Verification items for the finished model (mm, model axes). Give positions to 0.01 mm unless a question says otherwise; leave off trailing zeros. Write each loop counter-clockwise with the first axis right and the second up, starting at its lowest first coordinate (ties: lowest second). Pieces come first, ordered by that corner, then holes. Notation, with made-up numbers: M 25.5,78 L 35.5,78 A16 cw 35.5,98 Z; hole C -9.75,59.25 d7. An arc over 180 degrees is marked long. Write item = value, one per line.
from build123d import *

# Parameters (mm, degrees)
SKETCH3_W = 9
SKETCH3_H = 1.5


with BuildPart() as part:
    # Sweep1: sweep along a path in Sketch2
    with BuildLine(Plane.XY.offset(-150.483366658)) as sweep1_path:
        Line((-1, 148.379342702), (883.52063783, 148.379342702))
        ThreePointArc((883.52063783, 148.379342702), (890.42063783, 141.479342703), (883.52063783, 134.579342702))
        Line((883.52063783, 134.579342702), (-1, 134.579342702))
        ThreePointArc((-1, 134.579342702), (-7.9, 141.479342702), (-1, 148.379342702))
    # Sketch3 → Sweep1 (sweep)
    with BuildSketch(Plane(origin=(0, 0, 0), x_dir=(0, 0, -1), z_dir=(1, 0, 0))):
        with Locations((145.983366658, 147.629342702)):
            Rectangle(SKETCH3_W, SKETCH3_H)
    sweep(path=sweep1_path.line)


solid = part.part
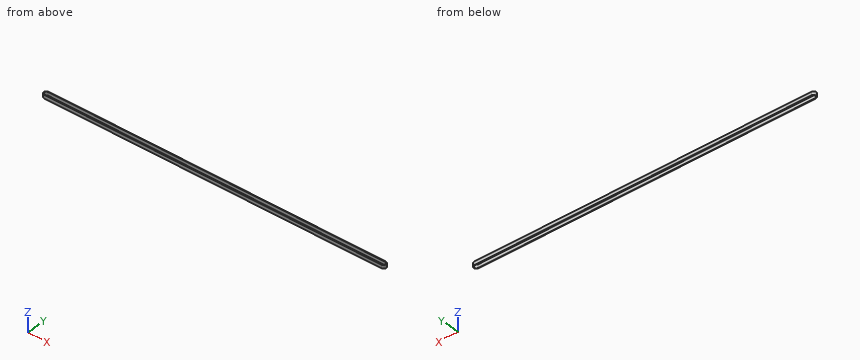
1) Depth check by flat-ended pin: P1, Ø1.5, axis at y = 142.5, z = -149.5, coming from the +X side; P2, Ø3, axis at y = 137, z = -147.5, coming from the -X side; P3, Ø1, axis at y = 146, z = -143.5, coming from the -X side. Enter the tip coordinate at first touch or a pass-through.
From the geometry:
P1 = 890.42
P2 = -7.22
P3 = -6.61
2) Cross-section at B-B on z = -145.5. Record the boundary of the cut face in (x, y).
From the geometry:
outline = M -1,134.58 L 883.52,134.58 A6.9 ccw 883.52,148.38 L -1,148.38 A6.9 ccw Z; hole M -1,136.08 L 883.52,136.08 A5.4 ccw 883.52,146.88 L -1,146.88 A5.4 ccw Z
3) Cross-section at A-A on x = 735. Record the boundary of the cut face in (y, z), plus the area to 3 significant figures.
From the geometry:
outline = M 134.58,-150.48 L 136.08,-150.48 L 136.08,-141.48 L 134.58,-141.48 Z; M 146.88,-150.48 L 148.38,-150.48 L 148.38,-141.48 L 146.88,-141.48 Z
area = 27.0 mm^2
4) Material ranges on probe 1 along Y at (x, z) = (614.5, -150); probe 2 along X at (y, z) = (142, -143); probe 3 along X at (y, z) = (140.5, -144.5), recorded low to high. Write a range as from..to.
From the geometry:
probe_1 = 134.58..136.08, 146.88..148.38
probe_2 = -7.88..-6.37, 888.9..890.4
probe_3 = -7.83..-6.31, 888.83..890.35
